from build123d import *

# Parameters (mm, degrees)
SKETCH1_W           = 127.635
SKETCH1_H           = 127.635
BOSS_EXTRUDE1_DEPTH = 9.525
SKETCH6_R           = 1.35255
F_6_32_HOLE1_DEPTH  = 12.7
SKETCH7_R           = 1.35255
F_6_32_HOLE2_DEPTH  = 12.7
SKETCH8_R           = 1.35255
F_6_32_HOLE3_DEPTH  = 12.7
SKETCH9_R           = 1.35255
F_6_32_HOLE4_DEPTH  = 12.7
SKETCH5_R           = 46.355
CUT_EXTRUDE1_DEPTH  = 9.525
SKETCH11_R          = 1.4351
CUT_EXTRUDE3_DEPTH  = 10.525
CIRPATTERN1_COUNT   = 12
SKETCH12_R          = 56.41975
CUT_EXTRUDE4_DEPTH  = 1.27


with BuildPart() as part:
    # Sketch1 → Boss-Extrude1 (new body)
    with BuildSketch(Plane(origin=(0, 0, 0), x_dir=(1, 0, 0), z_dir=(0, 1, 0))):
        with Locations((63.8175, 63.8175)):
            Rectangle(SKETCH1_W, SKETCH1_H)
    extrude(amount=BOSS_EXTRUDE1_DEPTH)

    # Sketch6 → 6-32 hole1 (cut)
    with BuildSketch(Plane(origin=(127.635, 0, 0), x_dir=(0, 0, -1), z_dir=(1, 0, 0))):
        with Locations((4.7625, 4.7625)):
            Circle(SKETCH6_R)
    extrude(amount=-F_6_32_HOLE1_DEPTH, mode=Mode.SUBTRACT)

    # Sketch7 → 6-32 hole2 (cut)
    with BuildSketch(Plane(origin=(0, 0, -127.635), x_dir=(-1, 0, 0), z_dir=(0, 0, -1))):
        with Locations((-122.8725, 4.7625)):
            Circle(SKETCH7_R)
    extrude(amount=-F_6_32_HOLE2_DEPTH, mode=Mode.SUBTRACT)

    # Sketch8 → 6-32 hole3 (cut)
    with BuildSketch(Plane.ZY):
        with Locations((-122.8725, 4.7625)):
            Circle(SKETCH8_R)
    extrude(amount=-F_6_32_HOLE3_DEPTH, mode=Mode.SUBTRACT)

    # Sketch9 → 6-32 hole4 (cut)
    with BuildSketch(Plane.XY):
        with Locations((4.7625, 4.7625)):
            Circle(SKETCH9_R)
    extrude(amount=-F_6_32_HOLE4_DEPTH, mode=Mode.SUBTRACT)

    # Sketch5 → Cut-Extrude1 (cut)
    with BuildSketch(Plane(origin=(0, 9.525, 0), x_dir=(1, 0, 0), z_dir=(0, 1, 0))):
        with Locations((63.8175, 63.8175)):
            Circle(SKETCH5_R)
    extrude(amount=-CUT_EXTRUDE1_DEPTH, mode=Mode.SUBTRACT)

    # Sketch11 → Cut-Extrude3 (cut, through all)
    with BuildSketch(Plane(origin=(0, 9.525, 0), x_dir=(1, 0, 0), z_dir=(0, 1, 0))):
        with Locations((63.8175, 115.443)):
            Circle(SKETCH11_R)
    cut_extrude3 = extrude(amount=-CUT_EXTRUDE3_DEPTH, mode=Mode.SUBTRACT)

    # CirPattern1: Cut-Extrude3 ×12 about axis
    cirpattern1_axis = Axis((63.8175, 0, -63.8175), (0, 1, 0))
    for i in range(1, CIRPATTERN1_COUNT):
        add(cut_extrude3.rotate(cirpattern1_axis, i * 360 / CIRPATTERN1_COUNT), mode=Mode.SUBTRACT)

    # Sketch12 → Cut-Extrude4 (cut)
    with BuildSketch(Plane(origin=(0, 9.525, 0), x_dir=(1, 0, 0), z_dir=(0, 1, 0))):
        with Locations((63.8175, 63.8175)):
            Circle(SKETCH12_R)
    extrude(amount=-CUT_EXTRUDE4_DEPTH, mode=Mode.SUBTRACT)


solid = part.part
Geometry: final body of the model. Coordinates: model frame, mm. A direction names the side the tool comes from. Round coordinates to 2 decimals unless told otherwise and drop trailing zeros. Order: outer loops, then holes, each group sorted by start corner. A loop starts at its lowest first (then second) coordinate and runs counter-clockwise, first axis right, second up.
Q1. Section C-C, the plane y = 1.75. Give the number of separate pieces and of enclosed holes in the cut face, and give its area (3 significant figures).
Result sheet:
separate pieces: 1
enclosed holes: 13
area: 9,460 mm2
Q2. Material intervals for probe 1 along Z at (x, y) = (64, 2.5) (3 decimals); probe 2 along Z at (x, y) = (39, 2.25) (3 decimals); probe 3 along X at (y, z) = (6.25, -105.5) (3 decimals), sorted ascending.
Result sheet:
probe 1: z = -127.635 to -116.866, -114.02 to -110.172, -17.463 to -13.615, -10.769 to 0
probe 2: z = -127.635 to -109.56, -107.493 to -102.969, -24.666 to -20.142, -18.075 to 0
probe 3: x = 0 to 43.536, 84.099 to 127.635
Q3. Section A-A, the plane z = -47. Output: boundary loops of the cut face in (x, y) (3 decimals).
Result sheet:
outline: (0, 0) - (20.621, 0) - (20.621, 8.255) - (9.963, 8.255) - (9.963, 9.525) - (0, 9.525) - close; (107.014, 0) - (127.635, 0) - (127.635, 9.525) - (117.672, 9.525) - (117.672, 8.255) - (107.014, 8.255) - close
Q4. Pin query (flat end, axial travel): pin 1 (2.5 mm diameter, centred on x = 19.11, z = -89.63, fed in from -Y); pin 2 (3.5 mm diameter, centred on x = 38, z = -19.11, fed in from +Y) (3 decimals). Return the tip coordinate at first contact, or that it passes through.
Result sheet:
pin 1: passes through
pin 2: stops at y = 8.255
Q5. Access query for faces 1 (the face through (43, 8.255, -22)), 2 (the face through (114.17, 4.185, -63.155)). Directions: +Z, -Z, +X, -X, +Y, -Y. A direction counts if a zero-diameter tool reaches every point of the face in a straight line with its end or side. Return the directions, or none.
Result sheet:
face 1: +Y
face 2: +Y, -Y
Q6. Section D-D, the plane x = 118.5. Output: boundary loops of the cut face in (y, z) (1 decimal).
Result sheet:
outline: (0, -127.6) - (9.5, -127.6) - (9.5, -77.7) - (8.3, -77.7) - (8.3, -49.9) - (9.5, -49.9) - (9.5, 0) - (0, 0) - close; hole circle Ø2.7 at (4.8, -4.8)
Q7. Section B-B, the plane x = 69.5. Output: boundary loops of the cut face in (y, z) (3 decimals), and give its area (3 significant figures).
Result sheet:
outline: (0, -127.635) - (9.525, -127.635) - (9.525, -119.95) - (8.255, -119.95) - (8.255, -109.823) - (0, -109.823) - close; (0, -17.812) - (8.255, -17.812) - (8.255, -7.685) - (9.525, -7.685) - (9.525, 0) - (0, 0) - close
area: 314 mm2
Q8. Mould query, pull axis Z, two halves, no side actions, for faces 3 (the face through (108.032, 4.185, -77.741)), 4 (the face through (63, 5, 0)), 5 (the face through (91, 0, -107)). Classes: released by +Z, released by -Z, zero draft, split by the parting line, or undercut.
Result sheet:
face 3: undercut
face 4: released by +Z
face 5: zero draft
